from build123d import *

# Parameters (mm, degrees)
SKETCH2_R          = 35
CUT_EXTRUDE1_DEPTH = 20
SKETCH3_W          = 70
SKETCH3_H          = 100
CUT_EXTRUDE2_DEPTH = 53


with BuildPart() as part:
    # Sketch1 → Revolve1 (revolve)
    with BuildSketch(Plane(origin=(0, 0, 0), x_dir=(1, 0, 0), z_dir=(0, 1, 0)), mode=Mode.PRIVATE) as revolve1_sk:
        with BuildLine():
            Line((35, 0), (-140, 0))
            Line((-140, 0), (-140, 42.5))
            Line((-140, 42.5), (1.859986247, 34.950542931))
            ThreePointArc((1.859986247, 34.950542931), (25.397829815, 24.082156064), (35, 0))
        make_face()
    revolve(revolve1_sk.sketch.rotate(Axis((35, 0, 0), (-1, 0, 0)), 180), axis=Axis((35, 0, 0), (-1, 0, 0)))

    # Sketch2 → Cut-Extrude1 (cut)
    with BuildSketch(Plane.ZY.offset(140)):
        Circle(SKETCH2_R)
    extrude(amount=-CUT_EXTRUDE1_DEPTH, mode=Mode.SUBTRACT)

    # Sketch3 → Cut-Extrude2 (cut)
    with BuildSketch(Plane.XY):
        Rectangle(SKETCH3_W, SKETCH3_H)
    extrude(amount=-CUT_EXTRUDE2_DEPTH, mode=Mode.SUBTRACT)

    # Sketch4 → Revolve2 (revolve)
    with BuildSketch(Plane.XY):
        with BuildLine():
            Line((25, 0), (-25, 0))
            ThreePointArc((-25, 0), (0, 25), (25, 0))
        make_face()
    revolve(axis=Axis((25, 0, 0), (-1, 0, 0)))


solid = part.part
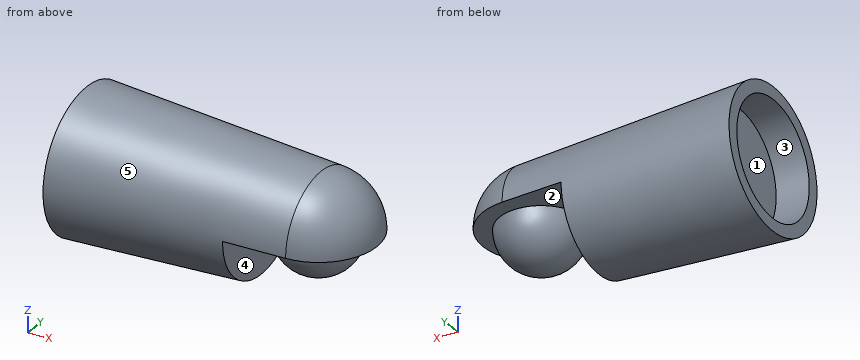
Build history of the part. All positions in model axes, mm. Face numbers are marked on the shaded views. A direction names the side the tool comes from. Give positions to 0.01 mm unless a question says otherwise; leave off trailing zeros. Write each loop counter-clockwise with the first axis right and the second up, starting at its lowest first coordinate (ties: lowest second). Pieces come first, ordered by that corner, then holes. Notation, with made-up numbers: (2.5, 25.25) - (18.5, 25.25) arc R11 cw to (18.5, 45.25) - close; hole circle Ø6 at (56.5, 45.25). An arc over 180 degrees is marked (long way). Use one line per item in the form item = value. Start each with the question number.
1. Band-saw the part on C-C on x = -73.5. Write the cut outline in (y, z).
2. Band-saw the part on B-B on x = -106. Write the cut outline in (y, z).
3. 3-axis set-ups, long thin cutter, end or side, ignore diameter. For the marked faces 1 and 2: which of +Z, -Z, +X, -X, +Y, -Y reach the whole face in a straight line?
4. Drop flat-ended pins along their axis: pin 1 Ø2 at (x, y) = (-95, 32) entering from +Z; pin 2 Ø4 at (x, z) = (8.5, 30) entering from +Y; pin 3 Ø21 at (y, z) = (10.5, -6) entering from -X. Give the stop position or say it passes through.
5. Band-saw the part on A-A on y = 0. Write the cut outline in (x, z).
6. Probe line 1 (X direction, y = 22, z = -28); line 2 (Y direction, x = -125, z = 0); line 3 (X direction, y = -25.5, z = -3). List the from-to ranges inside material, lowest first. Write a range as [from, to].
7. Two-plate mould, pull along Y, no slides. Class the marked faces 3, 4 and 5: released by +Y, released by -Y, zero draft, split by the parting line, or undercut.
Conclusion:
q1.outline = circle Ø77.92 at (0, 0)
q2.outline = circle Ø81.38 at (0, 0)
q3.face_1 = -X
q3.face_2 = -Z
q4.pin_1 = 25.45
q4.pin_2 = 19.33
q4.pin_3 = -120
q5.outline = (-140, -42.5) - (-35, -36.91) - (-35, 0) - (-25, 0) arc R25 ccw to (25, 0) - (35, 0) arc R35 ccw to (1.86, 34.95) - (-140, 42.5) - (-140, 35) - (-120, 35) - (-120, -35) - (-140, -35) - close
q6.line_1 = [-140, -35]
q6.line_2 = [-41.7, -35], [35, 41.7]
q6.line_3 = [-120, -35]
q7.face_3 = undercut
q7.face_4 = zero draft
q7.face_5 = split by the parting line
